Geometry check sheet. Reference: the model listing, model coordinates, mm. Face numbers are marked on the shaded views. A direction names the side the tool comes from. Coordinates: 2 decimals unless noted, no trailing zeros. Write each loop counter-clockwise with the first axis right and the second up, starting at its lowest first coordinate (ties: lowest second). Pieces come first, ordered by that corner, then holes. Notation, with made-up numbers: (59, 84) - (84, 84) arc R29 ccw to (84, 104) - close; hole circle Ø7 at (-20.75, 74). An arc over 180 degrees is marked (long way). Answer as a JSON object with one key per item and string values. Group by question number.
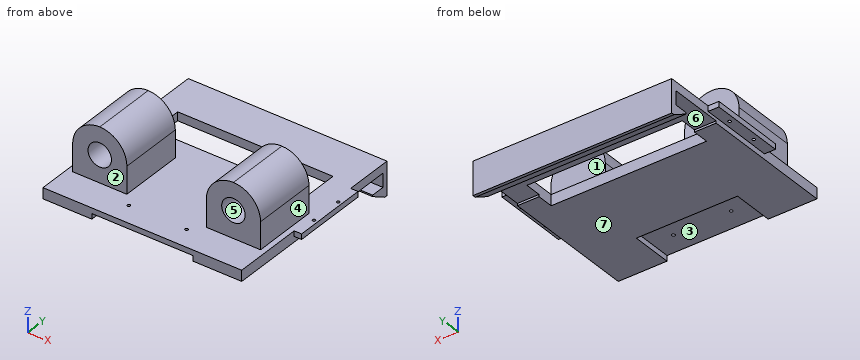
from build123d import *

# Parameters (mm, degrees)
CROQUIS1_W                 = 180
CROQUIS1_H                 = 180
SALIENTE_EXTRUIR1_DEPTH    = 30.7
CROQUIS2_W                 = 180
CROQUIS2_H                 = 162.21
CORTAR_EXTRUIR1_DEPTH      = 20.7
CROQUIS3_W                 = 10.7
CROQUIS3_H                 = 12.79
CORTAR_EXTRUIR2_DEPTH      = 274.7
SALIENTE_EXTRUIR2_DEPTH    = 20
CORTAR_EXTRUIR3_DEPTH      = 147
CORTAR_EXTRUIR3_DEPTH_BACK = 147
CROQUIS5_W                 = 10
CROQUIS5_H                 = 45
CROQUIS5_W_2               = 6.8
CROQUIS6_W                 = 93.2
CROQUIS6_H                 = 38
CROQUIS6_W_2               = 6.8
CROQUIS6_H_2               = 70
CROQUIS6_W_3               = 10
CORTAR_EXTRUIR4_DEPTH      = 5
CROQUIS7_W                 = 183.2
CROQUIS7_H                 = 50
CORTAR_EXTRUIR5_DEPTH      = 2
CROQUIS8_W                 = 45
CROQUIS8_H                 = 10
SALIENTE_EXTRUIR3_DEPTH    = 38
CROQUIS9_R                 = 1.4
CROQUIS9_W                 = 143.2
CROQUIS9_H                 = 30
CORTAR_EXTRUIR6_DEPTH      = 20
CHAFL_N1_SIZE              = 15
CHAFL_N1_SIZE2             = 8.660254038
CROQUIS10_W                = 50
CROQUIS10_H                = 60
SALIENTE_EXTRUIR4_DEPTH    = 50
REDONDEO1_R                = 25
CROQUIS11_R                = 10.8
CORTAR_EXTRUIR7_DEPTH      = 40


with BuildPart() as part:
    # Croquis1 → Saliente-Extruir1 (new body)
    with BuildSketch(Plane.XY):
        with Locations((90, 90)):
            Rectangle(CROQUIS1_W, CROQUIS1_H)
    extrude(amount=SALIENTE_EXTRUIR1_DEPTH)

    # Croquis2 → Cortar-Extruir1 (cut)
    with BuildSketch(Plane(origin=(0, 0, 0), x_dir=(-1, 0, 0), z_dir=(0, 0, -1))):
        with Locations((-90, 81.105)):
            Rectangle(CROQUIS2_W, CROQUIS2_H)
    extrude(amount=-CORTAR_EXTRUIR1_DEPTH, mode=Mode.SUBTRACT)

    # Croquis3 → Cortar-Extruir2 (cut)
    with BuildSketch(Plane.ZY):
        with Locations((15.35, 168.605)):
            Rectangle(CROQUIS3_W, CROQUIS3_H)
    extrude(amount=-CORTAR_EXTRUIR2_DEPTH, mode=Mode.SUBTRACT)

    # Croquis4 → Saliente-Extruir2 (add)
    with BuildSketch(Plane(origin=(180, 0, 0), x_dir=(0, 0, -1), z_dir=(1, 0, 0))):
        Polygon((-20.7, 0), (-20.7, 175), (-10, 175), (-10, 162.21), (0, 162.21), (0, 180), (-30.7, 180), (-30.7, 0), align=None)
    extrude(amount=SALIENTE_EXTRUIR2_DEPTH)

    # Croquis5 → Cortar-Extruir3 (cut, two sides: drawn at the far end of the back side and taken through both)
    with BuildSketch(Plane(origin=(0, 0, 20.7), x_dir=(-1, 0, 0), z_dir=(0, 0, -1)).offset(-CORTAR_EXTRUIR3_DEPTH_BACK)):
        Polygon((-55, 38), (-10, 38), (-10, 65), (0, 65), (0, 38), (0, 0), (-55, 0), align=None)
        Polygon((-148.2, 38), (-193.2, 38), (-193.2, 65), (-200, 65), (-200, 38), (-200, 0), (-148.2, 0), align=None)
        with Locations((-5, 157.5)):
            Rectangle(CROQUIS5_W, CROQUIS5_H)
        with Locations((-196.6, 157.5)):
            Rectangle(CROQUIS5_W_2, CROQUIS5_H)
    extrude(amount=CORTAR_EXTRUIR3_DEPTH + CORTAR_EXTRUIR3_DEPTH_BACK, mode=Mode.SUBTRACT)

    # Croquis6 → Cortar-Extruir4 (cut)
    with BuildSketch(Plane(origin=(0, 0, 20.7), x_dir=(-1, 0, 0), z_dir=(0, 0, -1))):
        with Locations((-101.6, 19)):
            Rectangle(CROQUIS6_W, CROQUIS6_H)
        with Locations((-196.6, 100)):
            Rectangle(CROQUIS6_W_2, CROQUIS6_H_2)
        with Locations((-5, 100)):
            Rectangle(CROQUIS6_W_3, CROQUIS6_H_2)
    extrude(amount=-CORTAR_EXTRUIR4_DEPTH, mode=Mode.SUBTRACT)

    # Croquis7 → Cortar-Extruir5 (cut)
    with BuildSketch(Plane(origin=(0, 0, 20.7), x_dir=(-1, 0, 0), z_dir=(0, 0, -1))):
        with Locations((-101.6, 150)):
            Rectangle(CROQUIS7_W, CROQUIS7_H)
    extrude(amount=-CORTAR_EXTRUIR5_DEPTH, mode=Mode.SUBTRACT)

    # Croquis8 → Saliente-Extruir3 (add)
    with BuildSketch(Plane.XZ.offset(-38)):
        with Locations((32.5, 25.7)):
            Rectangle(CROQUIS8_W, CROQUIS8_H)
        with Locations((170.7, 25.7)):
            Rectangle(CROQUIS8_W, CROQUIS8_H)
    extrude(amount=SALIENTE_EXTRUIR3_DEPTH)

    # Croquis9 → Cortar-Extruir6 (cut)
    with BuildSketch(Plane.XY.offset(30.7)):
        with Locations((5, 115)):
            Circle(CROQUIS9_R)
        with Locations((5, 85)):
            Circle(CROQUIS9_R)
        with Locations((196.6, 115)):
            Circle(CROQUIS9_R)
        with Locations((196.6, 85)):
            Circle(CROQUIS9_R)
        with Locations((128.2, 19)):
            Circle(CROQUIS9_R)
        with Locations((75, 19)):
            Circle(CROQUIS9_R)
        with Locations((101.6, 125)):
            Rectangle(CROQUIS9_W, CROQUIS9_H)
    extrude(amount=-CORTAR_EXTRUIR6_DEPTH, mode=Mode.SUBTRACT)

    # Chaflán1
    chafl_n1_edges = [part.edges().sort_by_distance(p)[0] for p in [
        (101.6, 162.21, 0),
    ]]
    chafl_n1_side = [part.faces().sort_by_distance(p)[0] for p in [
        (101.6, 171.105, 0),
    ]]
    chamfer(chafl_n1_edges, length=CHAFL_N1_SIZE, length2=CHAFL_N1_SIZE2, reference=chafl_n1_side[0])

    # Croquis10 → Saliente-Extruir4 (add)
    with BuildSketch(Plane.XY.offset(30.7)):
        with Locations((163.2, 60)):
            Rectangle(CROQUIS10_W, CROQUIS10_H)
        with Locations((40, 60)):
            Rectangle(CROQUIS10_W, CROQUIS10_H)
    extrude(amount=SALIENTE_EXTRUIR4_DEPTH)

    # Redondeo1
    redondeo1_edges = [part.edges().sort_by_distance(p)[0] for p in [
        (15, 60, 80.7),
        (65, 60, 80.7),
        (138.2, 60, 80.7),
        (188.2, 60, 80.7),
    ]]
    fillet(redondeo1_edges, radius=REDONDEO1_R - 0.0001)  # a hair under: the kernel refuses the full size

    # Croquis11 → Cortar-Extruir7 (cut)
    with BuildSketch(Plane.XZ.offset(-30)):
        with Locations(Location((163.2, 55.7, 0), (0, 0, 270))):
            Circle(CROQUIS11_R)
        with Locations(Location((40, 55.7, 0), (0, 0, 270))):
            Circle(CROQUIS11_R)
    extrude(amount=-CORTAR_EXTRUIR7_DEPTH, mode=Mode.SUBTRACT)


solid = part.part
(1) Draft check along Z on the marked faces 4, 5, 6 and 7. Enter one of: +Z half, -Z half, draft (parallel to the pull), parting line (faces both ways), or undercut.
(2) Gauge pin test, flat ends, axial feed: pin 1 (1.5 mm diameter, centred on x = 89, z = 9, fed in from -Y); pin 2 (8 mm diameter, centred on y = 67, z = 47.5, fed in from +X); pin 3 (4 mm diameter, centred on x = 34, y = 108, fed in from -Z). Record the tip position at first contact, or that the pin passes through.
(3) Section check A-A (z = 35.5). Record the cut outline in (x, y).
(4) Material ranges on L1, parallel to X at y = 115, z = 27.5; L2, parallel to X at y = 48, z = 55.7; L3, parallel to X at y = 85, z = 28, recorded low to high. Write a range as [from, to].
(5) Section check C-C (y = 100). Record the cut outline in (x, z), and give its area (3 significant figures).
(6) Section check D-D (z = 51.5). Record the cut outline in (x, y), and give its area (3 significant figures).
(7) Section check B-B (y = 120). Record the cut outline in (x, z), and give its area (3 significant figures).
(8) Set-up check for the marked faces 1, 2 and 3: record each of +Z, -Z, +X, -X, +Y, -Y from which the full face is reachable in a straight line by a thin tool's end or side.
Conclusion:
{
 "1": {"face 4": "draft", "face 5": "undercut", "face 6": "undercut", "face 7": "-Z half"},
 "2": {"pin 1": "stops at y = 162.21", "pin 2": "stops at x = 188.2", "pin 3": "stops at z = 20.7"},
 "3": {"outline": "(15, 30) - (65, 30) - (65, 90) - (15, 90) - close; (138.2, 30) - (188.2, 30) - (188.2, 90) - (138.2, 90) - close"},
 "4": {"L1": "x = [0, 3.6], [6.4, 30], [173.2, 195.2], [198, 200]", "L2": "x = [15, 29.2], [50.8, 65], [138.2, 152.4], [174, 188.2]", "L3": "x = [0, 3.6], [6.4, 195.2], [198, 200]"},
 "5": {"outline": "(0, 25.7) - (10, 25.7) - (10, 20.7) - (193.2, 20.7) - (193.2, 25.7) - (200, 25.7) - (200, 30.7) - (0, 30.7) - close", "area": "1,920 mm^2"},
 "6": {"outline": "(15, 30) - (30.05, 30) - (30.05, 70) - (49.95, 70) - (49.95, 30) - (65, 30) - (65, 90) - (15, 90) - close; (138.2, 30) - (153.25, 30) - (153.25, 70) - (173.15, 70) - (173.15, 30) - (188.2, 30) - (188.2, 90) - (138.2, 90) - close", "area": "4,410 mm^2"},
 "7": {"outline": "(0, 25.7) - (10, 25.7) - (10, 20.7) - (30, 20.7) - (30, 30.7) - (0, 30.7) - close; (173.2, 20.7) - (193.2, 20.7) - (193.2, 25.7) - (200, 25.7) - (200, 30.7) - (173.2, 30.7) - close", "area": "484 mm^2"},
 "8": {"face 1": "+Z, +X, -X, +Y", "face 2": "+Z, +X, -X, -Y", "face 3": "-Z, -Y"}
}
